Design review of the part shown in the three views and the two pictorial views. Dimensions are in mm from the part's minimum x, y and z. Coordinates: 2 decimals unless noted, no trailing zeros. Write each loop counter-clockwise with the first axis right and the second up, starting at its lowest first coordinate (ties: lowest second). Pieces come first, ordered by that corner, then holes. Notation, with made-up numbers: (0.25, 82.5) - (14.25, 82.5) arc R25 cw to (14.25, 95.5) - close; hole circle Ø2 at (66.25, 75). An arc over 180 degrees is marked (long way). Return JSON: item names as keys, results as strings. Group by question number.
(1) We need section B-B on x = 1.75. State the section outline as (y, z) points, then the cut area to 3 significant figures.
(2) We need section C-C on y = 1.5. State the section outline as (x, z) points.
(3) For pin 1 Ø3 at (y, z) = (4.5, 3.5) entering from -X; pin 2 Ø1.5 at (y, z) = (7.5, 14) entering from +X; pin 3 Ø1.5 at (x, y) = (12, 7) entering from -Z, all flat-tipped, find the tip position at first contact; note any pin that passes through.
(4) We need section A-A on z = 14.5. State the section outline as (x, y) points.
(5) To check wall thickness, follow L1, parallel to X at y = 7.25, z = 8; L2, parallel to Z at x = 7.5, y = 5.5; L3, parallel to Z at x = 1, y = 9.5. State the ranges of each line that lie inside material, in increasing order. Write a range as from..to.
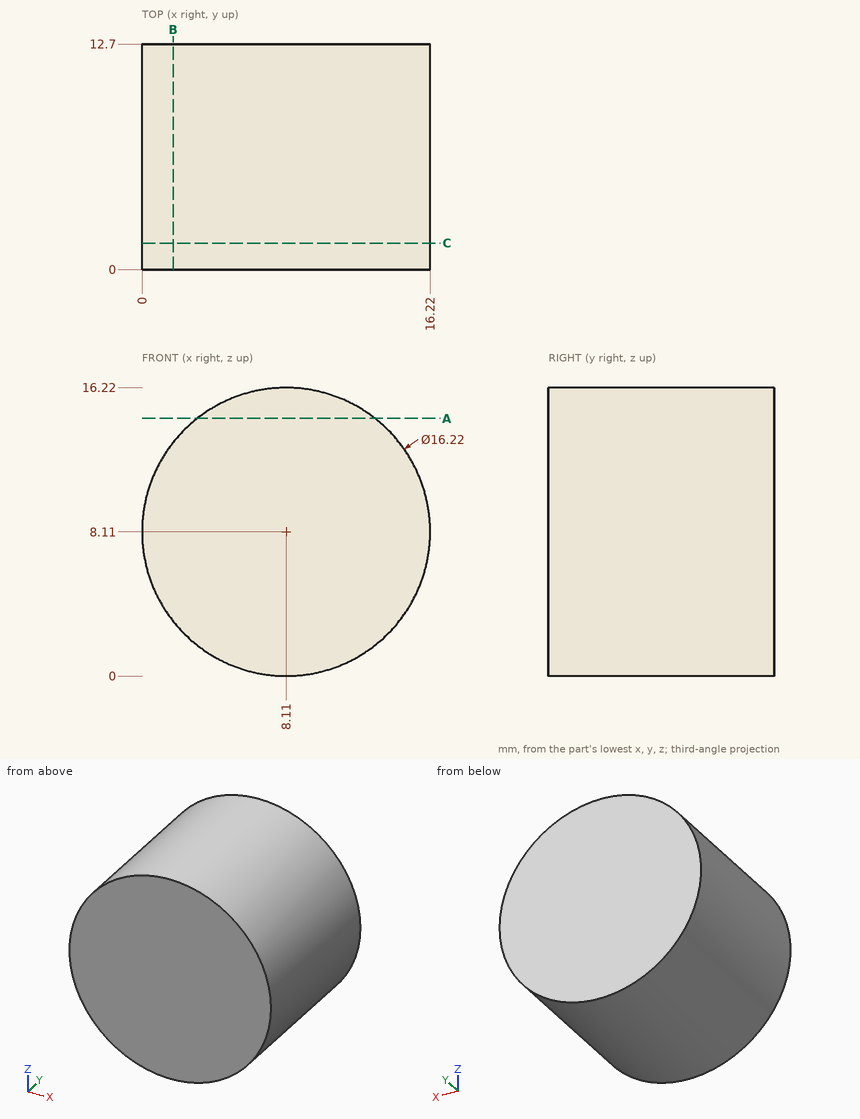
Ans:
{
 "1": {"outline": "(0, 3.08) - (12.7, 3.08) - (12.7, 13.14) - (0, 13.14) - close", "area": "128 mm²"},
 "2": {"outline": "circle Ø16.22 at (8.11, 8.11)"},
 "3": {"pin 1": "x = 0.62", "pin 2": "x = 14.38", "pin 3": "z = 0.63"},
 "4": {"outline": "(3.12, 0) - (13.1, 0) - (13.1, 12.7) - (3.12, 12.7) - close"},
 "5": {"L1": "0..16.22", "L2": "0.02..16.2", "L3": "4.21..12.01"}
}
